The model under review builds one solid part; all positions refer to its coordinate system, in mm. A direction names the side the tool comes from. Coordinates: 2 decimals unless noted, no trailing zeros.
```python
from build123d import *

# Parameters (mm, degrees)
F0_W           = 30
F0_H           = 30
F1_DEPTH       = 30
F2_R           = 2.5
F8_D           = 3
F8_DEPTH       = 1
F8_TIP         = 0.9012909285
F8_ON_F4_D     = 3
F8_ON_F4_DEPTH = 1
F8_ON_F4_TIP   = 0.9012909285
F8_ON_F7_D     = 3
F8_ON_F7_DEPTH = 1
F8_ON_F7_TIP   = 0.9012909285
F8_ON_F6_D     = 3
F8_ON_F6_DEPTH = 1
F8_ON_F6_TIP   = 0.9012909285
F8_ON_F5_D     = 3
F8_ON_F5_DEPTH = 1
F8_ON_F5_TIP   = 0.9012909285


with BuildPart() as f1:
    # F0 (on Front) → F1 (new body)
    with BuildSketch(Plane.XZ):
        Rectangle(F0_W, F0_H)
    extrude(amount=F1_DEPTH)

    # F2
    f2_edges = [f1.edges().sort_by_distance(p)[0] for p in [
        (15, -30, 0),
        (0, -30, 15),
        (-15, -30, 0),
        (0, -30, -15),
        (15, -15, 15),
        (-15, -15, 15),
        (0, 0, 15),
        (15, -15, -15),
        (15, 0, 0),
        (-15, -15, -15),
        (-15, 0, 0),
        (0, 0, -15),
    ]]
    fillet(f2_edges, radius=F2_R)

    # F8
    with Locations(Plane.XZ.offset(30)):
        with Locations((-5, 5), (5, 5), (5, 0), (-5, 0), (-5, -5), (5, -5)):
            Hole(F8_D / 2, depth=F8_DEPTH)
            with Locations((0, 0, -(F8_DEPTH + F8_TIP / 2))):  # 118° drill point
                Cone(0, F8_D / 2, F8_TIP, mode=Mode.SUBTRACT)

    # F8 on F4
    with Locations(Plane.XY.offset(15)):
        with Locations((-5, -20), (-5, -10), (5, -10), (5, -20)):
            Hole(F8_ON_F4_D / 2, depth=F8_ON_F4_DEPTH)
            with Locations((0, 0, -(F8_ON_F4_DEPTH + F8_ON_F4_TIP / 2))):  # 118° drill point
                Cone(0, F8_ON_F4_D / 2, F8_ON_F4_TIP, mode=Mode.SUBTRACT)

    # F8 on F7
    with Locations(Plane.YZ.offset(15)):
        with Locations((-10, 5), (-20, -5)):
            Hole(F8_ON_F7_D / 2, depth=F8_ON_F7_DEPTH)
            with Locations((0, 0, -(F8_ON_F7_DEPTH + F8_ON_F7_TIP / 2))):  # 118° drill point
                Cone(0, F8_ON_F7_D / 2, F8_ON_F7_TIP, mode=Mode.SUBTRACT)

    # F8 on F6
    with Locations(Plane(origin=(-15, 0, 0), x_dir=(0, -1, 0), z_dir=(-1, 0, 0))):
        with Locations((20.8823522035, 5), (15.8823522035, 0), (10.8823522035, -5), (10.8823522035, 5), (20.8823522035, -5)):
            Hole(F8_ON_F6_D / 2, depth=F8_ON_F6_DEPTH)
            with Locations((0, 0, -(F8_ON_F6_DEPTH + F8_ON_F6_TIP / 2))):  # 118° drill point
                Cone(0, F8_ON_F6_D / 2, F8_ON_F6_TIP, mode=Mode.SUBTRACT)

    # F8 on F5
    with Locations(Plane(origin=(0, 0, -15), x_dir=(1, 0, 0), z_dir=(0, 0, -1))):
        with Locations((-5, 10), (0, 15), (5, 20)):
            Hole(F8_ON_F5_D / 2, depth=F8_ON_F5_DEPTH)
            with Locations((0, 0, -(F8_ON_F5_DEPTH + F8_ON_F5_TIP / 2))):  # 118° drill point
                Cone(0, F8_ON_F5_D / 2, F8_ON_F5_TIP, mode=Mode.SUBTRACT)


solid = f1.part
```
(1) Machinability: for faces 1 (the face through (1.11, -16.01, -14.49)), 2 (the face through (-6.386, -29.493, 4.425)), 3 (the face through (-5.69, -11.33, 14.49)), which of the approach directions +Z, -Z, +X, -X, +Y, -Y give a long, thin tool a straight path to every point of the face, cutting with its end or side? Answer none if there is none.
A:
face 1: -Z
face 2: -Y
face 3: +Z
(2) Wall thickness on probe 1 along Z at (x, y) = (5, -29.5); probe 2 along Z at (x, y) = (-5, -29.4); probe 3 along X at (y, z) = (-10, 14.4): over which ranges is each line inside the solid? List them lowest first.
A:
probe 1: z = -14 to -6.5, -3.5 to -1.5, 1.5 to 3.5, 6.5 to 14
probe 2: z = -14.12 to -6.5, -3.5 to -1.5, 1.5 to 3.5, 6.5 to 14.12
probe 3: x = -14.12 to -6.5, -3.5 to 3.5, 6.5 to 14.12
(3) Draft analysis for pull direction Y (two halves, no side actions). For faces 4 (the face through (5.14, -19.78, 13.255)), 5 (the face through (-13.255, -10.676, -5.159)), 6 (the face through (0.175, -0.752, -14.287)), 7 (the face through (-14.287, -15.175, 14.248)), state which applies: released by +Y, released by -Y, zero draft, split by the parting line, or undercut.
A:
face 4: undercut
face 5: undercut
face 6: released by +Y
face 7: zero draft
(4) For pin 1 Ø1.8 at (x, y) = (-5, -10) entering from -Z, flat-tipped, find the tip position at first contact; note if it passes through.
A:
pin 1: stops at z = -13.64
